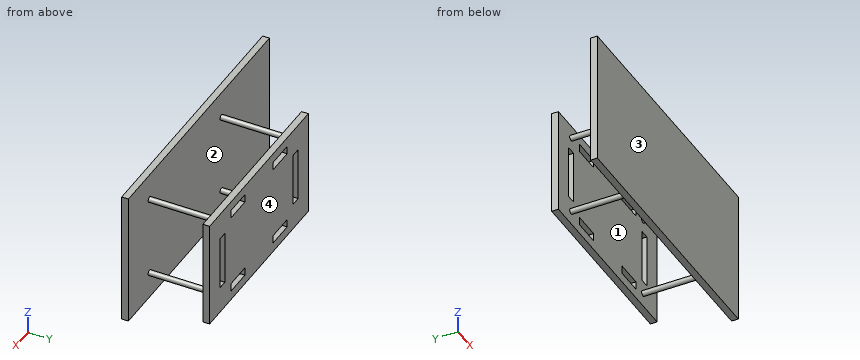
from build123d import *

# Parameters (mm, degrees)
SKETCH1_W           = 200
SKETCH1_H           = 100
BOSS_EXTRUDE2_DEPTH = 5
SKETCH2_R           = 2
BOSS_EXTRUDE3_DEPTH = 50
SKETCH3_W           = 140
SKETCH3_H           = 80
BOSS_EXTRUDE4_DEPTH = 5
SKETCH4_W           = 20
SKETCH4_H           = 6
CUT_EXTRUDE1_DEPTH  = 5
SKETCH7_W           = 7
SKETCH7_H           = 40
CUT_EXTRUDE2_DEPTH  = 5


with BuildPart() as part:
    # Sketch1 → Boss-Extrude2 (new body)
    with BuildSketch(Plane(origin=(0, 0, 0), x_dir=(1, 0, 0), z_dir=(0, 1, 0))):
        Rectangle(SKETCH1_W, SKETCH1_H)
    extrude(amount=BOSS_EXTRUDE2_DEPTH)

    # Sketch2 → Boss-Extrude3 (add)
    with BuildSketch(Plane(origin=(0, 5, 0), x_dir=(1, 0, 0), z_dir=(0, 1, 0))):
        with Locations((70, -30)):
            Circle(SKETCH2_R)
        with Locations((-32, -30)):
            Circle(SKETCH2_R)
        with Locations((70, 30)):
            Circle(SKETCH2_R)
        with Locations((-32, 30)):
            Circle(SKETCH2_R)
    extrude(amount=BOSS_EXTRUDE3_DEPTH)

    # Sketch3 → Boss-Extrude4 (add)
    with BuildSketch(Plane(origin=(0, 55, 0), x_dir=(1, 0, 0), z_dir=(0, 1, 0))):
        with Locations((20, 0)):
            Rectangle(SKETCH3_W, SKETCH3_H)
    extrude(amount=BOSS_EXTRUDE4_DEPTH)

    # Sketch4 → Cut-Extrude1 (cut)
    with BuildSketch(Plane(origin=(0, 60, 0), x_dir=(1, 0, 0), z_dir=(0, 1, 0))):
        with Locations((-10, 30)):
            Rectangle(SKETCH4_W, SKETCH4_H)
        with Locations((-10, -30)):
            Rectangle(SKETCH4_W, SKETCH4_H)
        with Locations((50, -30)):
            Rectangle(SKETCH4_W, SKETCH4_H)
        with Locations((50, 30)):
            Rectangle(SKETCH4_W, SKETCH4_H)
    extrude(amount=-CUT_EXTRUDE1_DEPTH, mode=Mode.SUBTRACT)

    # Sketch7 → Cut-Extrude2 (cut)
    with BuildSketch(Plane(origin=(0, 60, 0), x_dir=(1, 0, 0), z_dir=(0, 1, 0))):
        with Locations((-32, 0)):
            Rectangle(SKETCH7_W, SKETCH7_H)
        with Locations((72, 0)):
            Rectangle(SKETCH7_W, SKETCH7_H)
    extrude(amount=-CUT_EXTRUDE2_DEPTH, mode=Mode.SUBTRACT)


solid = part.part
Design review of the part built by this model. Coordinates are the model's own, in mm. Face numbers are marked on the shaded views. Coordinates: 2 decimals unless noted, no trailing zeros. Order: outer loops, then holes, each group sorted by start corner. A loop starts at its lowest first (then second) coordinate and runs counter-clockwise, first axis right, second up. Notation, with made-up numbers: (64, 23) - (100, 23) arc R30 ccw to (100, 51) - close; hole circle Ø4 at (23, -40). An arc over 180 degrees is marked (long way). Put each result on its own line as item: value.
1) Take a section at A-A, the plane z = 12. Give the boundary of the cut face in (x, y), and give its area (3 significant figures).
Response values:
outline: (-100, 0) - (100, 0) - (100, 5) - (-100, 5) - close; (-50, 55) - (-35.5, 55) - (-35.5, 60) - (-50, 60) - close; (-28.5, 55) - (68.5, 55) - (68.5, 60) - (-28.5, 60) - close; (75.5, 55) - (90, 55) - (90, 60) - (75.5, 60) - close
area: 1,630 mm²
2) The part is to be moulded in two halves that separate along Y. For the marked faces 1, 2, 3 and 4, say which applies: released by +Y, released by -Y, zero draft, split by the parting line, or undercut.
Response values:
face 1: undercut
face 2: undercut
face 3: released by -Y
face 4: released by +Y
3) Wall thickness on L1, parallel to Y at x = 3, z = -18.5; L2, parallel to Z at x = 70, y = 13; L3, parallel to Y at x = -69.5, z = 24: over which ranges is each line inside the solid? List them lowest first. Write a range as from..to.
Response values:
L1: y = 0..5, 55..60
L2: z = -32..-28, 28..32
L3: y = 0..5
4) Take a section at C-C, the plane z = -30. Give the boundary of the cut face in (x, y), and give its area (3 significant figures).
Response values:
outline: (-100, 0) - (100, 0) - (100, 5) - (72, 5) - (72, 55) - (90, 55) - (90, 60) - (60, 60) - (60, 55) - (68, 55) - (68, 5) - (-30, 5) - (-30, 55) - (-20, 55) - (-20, 60) - (-50, 60) - (-50, 55) - (-34, 55) - (-34, 5) - (-100, 5) - close; (0, 55) - (40, 55) - (40, 60) - (0, 60) - close
area: 1,900 mm²
5) Take a section at D-D, the plane y = 35.5. Give the boundary of the cut face in (x, z).
Response values:
outline: circle Ø4 at (-32, -30); circle Ø4 at (-32, 30); circle Ø4 at (70, -30); circle Ø4 at (70, 30)
6) Take a section at B-B, the plane x = 10.5. Give the boundary of the cut face in (y, z), and give its area (3 significant figures).
Response values:
outline: (0, -50) - (5, -50) - (5, 50) - (0, 50) - close; (55, -40) - (60, -40) - (60, 40) - (55, 40) - close
area: 900 mm²
7) Insertion check: P1, Ø6, axis at y = 32.5, z = -29.5, coming from the -X side; P2, Ø4, axis at y = 58, z = -29.5, coming from the +X side; P3, Ø4, axis at y = 57.5, z = 31, coming from the -X side. Each pin has a flat end and moves straight along its axis. Give the tip position at first contact, or say it passes through.
Response values:
P1: stops at x = -34
P2: stops at x = 90
P3: stops at x = -50
